Work out the finished part from the listing and answer in its coordinate system (mm). Face numbers are marked on the shaded views. A direction names the side the tool comes from. Give positions to 0.01 mm unless a question says otherwise; leave off trailing zeros. Write each loop counter-clockwise with the first axis right and the second up, starting at its lowest first coordinate (ties: lowest second). Pieces come first, ordered by that corner, then holes.
1) Find section A-A (x = 5.5). Determine the outline of the cut face in (y, z).
2) Find section B-B (y = 34). Determine the outline of the cut face in (x, z), plus the area to 3 significant figures.
3) Determine the mould class of the marked faces 1, 2 and 3 for opening direction Y: pulls with the +Y half, pulls with the -Y half, needs draft (parallel to the pull), parting line crosses it, or undercut.
4) Given pin 1 Ø13.5 at (x, y) = (12, -4.5) entering from +Z; pin 2 Ø11.5 at (x, y) = (18, 3.5) entering from +Z; pin 3 Ø6 at (x, y) = (14.5, 19.5) entering from +Z; pin 4 Ø1.5 at (y, z) = (40.5, -38) entering from -X, each flat-ended and moving along its own axis, determine where each tip first touches the part or whether it passes through.
5) Straight lines are drawn through the part: probe 1 along Y at (x, z) = (9.75, -21); probe 2 along Y at (x, z) = (16, -52); probe 3 along Z at (x, y) = (8.75, 30). For each, find the intervals that lie inside material, in ascending order.
6) Find section C-C (z = -45). Determine the outline of the cut face in (x, y), plus the area to 3 significant figures.
7) A tool of negligible diameter and unlimited length cuts with its end or side. For the marked faces 4 and 5, from which of +Z, -Z, +X, -X, +Y, -Y can it reach the whole face along a straight path? Write none if from no direction.
8) Find section D-D (y = -2). Determine the outline of the cut face in (x, z), plus the area to 3 significant figures.
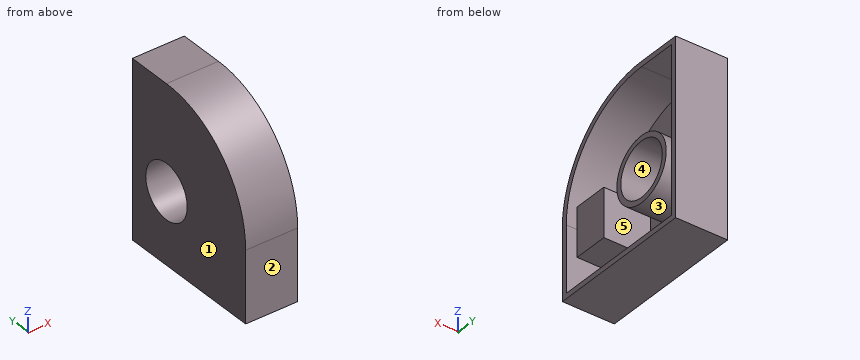
```python
from build123d import *

# Parameters (mm, degrees)
F0_W     = 72.689131
F0_H     = 85.548859
F1_DEPTH = 25.4
F2_R     = 50.8
F3_R     = 13.311226
F4_DEPTH = 25.4
F5_T     = -2.54
F6_W     = 17.114856
F6_H     = 23.744739
F7_DEPTH = 25.4


with BuildPart() as f1:
    # F0 (on Right) → F1 (new body)
    with BuildSketch(Plane.YZ):
        with Locations((15.549161, -12.564396)):
            Rectangle(F0_W, F0_H)
    extrude(amount=F1_DEPTH)

    # F2
    f2_edges = [f1.edges().sort_by_distance(p)[0] for p in [
        (12.7, -20.795405, 30.210033),
    ]]
    fillet(f2_edges, radius=F2_R)

    # F3 (on face) → F4 (cut)
    with BuildSketch(Plane.YZ.offset(25.4)):
        with Locations((30.004595, -20.589967)):
            Circle(F3_R)
    extrude(amount=-F4_DEPTH, mode=Mode.SUBTRACT)

    # F5
    f5_openings = [f1.faces().sort_by_distance(p)[0] for p in [
        (25.4, 16.684078, -15.097146),
    ]]
    offset(amount=F5_T, openings=f5_openings)

    # F6 (on Right) → F7 (join)
    with BuildSketch(Plane.YZ):
        with Locations((-2.747506, -27.793449)):
            Rectangle(F6_W, F6_H)
    extrude(amount=F7_DEPTH)


solid = f1.part
```
Results:
1. outline: (-20.8, -55.34) - (51.89, -55.34) - (51.89, 30.21) - (30, 30.21) arc R50.8 ccw to (-20.8, -20.59) - close; (-11.3, -39.67) - (5.81, -39.67) - (5.81, -15.92) - (-11.3, -15.92) - close; circle Ø31.7 at (30, -20.59); hole (-18.26, -52.8) - (49.35, -52.8) - (49.35, 27.67) - (30, 27.67) arc R48.26 ccw to (-18.26, -20.59) - close; hole circle Ø26.62 at (30, -20.59)
2. outline: (0, -55.34) - (25.4, -55.34) - (25.4, -52.8) - (2.54, -52.8) - (2.54, -35.93) - (25.4, -35.93) - (25.4, -33.29) - (0, -33.29) - close; (0, -7.89) - (25.4, -7.89) - (25.4, -5.25) - (2.54, -5.25) - (2.54, 27.67) - (25.4, 27.67) - (25.4, 30.21) - (0, 30.21) - close
2. area: 390 mm2
3. face 1: needs draft
3. face 2: pulls with the -Y half
3. face 3: undercut
4. pin 1: stops at z = 21.96
4. pin 2: stops at z = 25.78
4. pin 3: stops at z = 29.65
4. pin 4: stops at x = 0
5. probe 1: y = -20.8 to -18.26, -11.3 to 5.81, 14.16 to 16.7, 43.31 to 45.85, 49.35 to 51.89
5. probe 2: y = -20.8 to -18.26, 49.35 to 51.89
5. probe 3: z = -55.34 to -52.8, -36.44 to -33.9, -7.28 to -4.74, 27.67 to 30.21
6. outline: (0, -20.8) - (25.4, -20.8) - (25.4, -18.26) - (2.54, -18.26) - (2.54, 49.35) - (25.4, 49.35) - (25.4, 51.89) - (0, 51.89) - close
6. area: 301 mm2
7. face 4: +X, -X
7. face 5: +X
8. outline: (0, -55.34) - (25.4, -55.34) - (25.4, -52.8) - (2.54, -52.8) - (2.54, -39.67) - (25.4, -39.67) - (25.4, -15.92) - (2.54, -15.92) - (2.54, 15.53) - (25.4, 15.53) - (25.4, 18.86) - (0, 18.86) - close
8. area: 865 mm2
